Drawing for the job (mm, zero at the part's lowest x, y, z). Round coordinates to 2 decimals unless told otherwise and drop trailing zeros. Loops run counter-clockwise (first coordinate to the right, second up) from the corner with the lowest first, then second, coordinate; pieces in that order, holes last. Notation, with made-up numbers: (-2, 38.5) -> (4, 38.5) arc R17 cw to (4, 42.5) -> close; hole circle Ø10 at (-34, 38.5). An arc over 180 degrees is marked (long way). Put each result on its own line as item: value. Start each with the question number.
Item 1: Cut at B-B, the plane z = 6.5. List the corners of the cut face in (x, y).
Item 2: Flat gauge pins, fed straight in: pin 1 Ø1.5 at (x, z) = (121.5, 5) entering from -Y; pin 2 Ø1.5 at (y, z) = (2, 4) entering from -X; pin 3 Ø5 at (x, z) = (84.5, 3.5) entering from +Y. Where does each tip first touch, or does it go through?
Item 3: Drill centre lines: probe 1 along Y at (x, z) = (40, 5.75); probe 2 along X at (y, z) = (76, 8); probe 3 along Y at (x, z) = (104.5, 8). Where is each one in solid material? Low to high. Write a range as [from, to].
Item 4: Cut at C-C, the plane x = 63.5. List the corners of the cut face in (y, z), plus the area to 3 significant figures.
Item 5: Cut at A-A, the plane y = 73. List the corners of the cut face in (x, z).
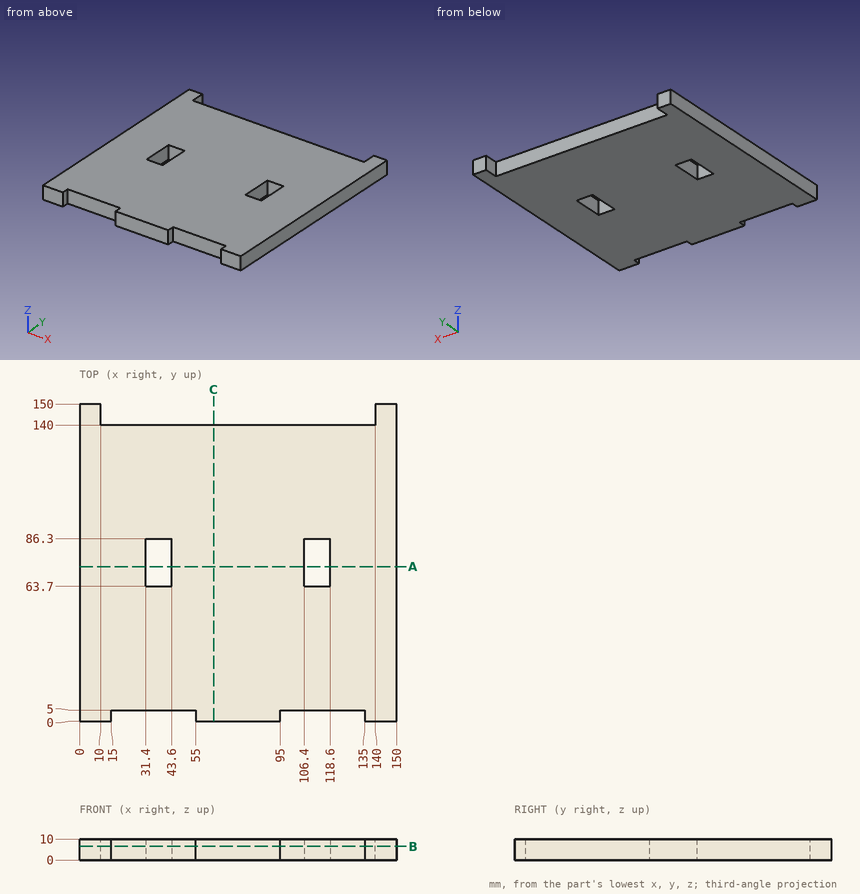
Reply:
1. outline: (0, 0) -> (15, 0) -> (15, 5) -> (55, 5) -> (55, 0) -> (95, 0) -> (95, 5) -> (135, 5) -> (135, 0) -> (150, 0) -> (150, 150) -> (140, 150) -> (140, 140) -> (10, 140) -> (10, 150) -> (0, 150) -> close; hole (31.4, 63.7) -> (43.6, 63.7) -> (43.6, 86.3) -> (31.4, 86.3) -> close; hole (106.4, 63.7) -> (118.6, 63.7) -> (118.6, 86.3) -> (106.4, 86.3) -> close
2. pin 1: stops at y = 5
2. pin 2: stops at x = 0
2. pin 3: stops at y = 140
3. probe 1: y = [5, 63.7], [86.3, 140]
3. probe 2: x = [0, 31.4], [43.6, 106.4], [118.6, 150]
3. probe 3: y = [5, 140]
4. outline: (0, 0) -> (140, 0) -> (140, 10) -> (0, 10) -> close
4. area: 1,400 mm^2
5. outline: (0, 0) -> (31.4, 0) -> (31.4, 10) -> (0, 10) -> close; (43.6, 0) -> (106.4, 0) -> (106.4, 10) -> (43.6, 10) -> close; (118.6, 0) -> (150, 0) -> (150, 10) -> (118.6, 10) -> close
